Could you check a few things on this model? Use its own coordinates, in mm. A direction names the side the tool comes from. Coordinates: 2 decimals unless noted, no trailing zeros. Loops run counter-clockwise (first coordinate to the right, second up) from the corner with the lowest first, then second, coordinate; pieces in that order, holes last.
from build123d import *

# Parameters (mm, degrees)
F1_DEPTH = 8


with BuildPart() as f1:
    # F0 (on Front) → F1 (new body)
    with BuildSketch(Plane.XZ):
        Polygon((10.056205, -4.107465), (10.056205, -7.790019), (3.824189, -7.790019), (3.824189, -11.472573), (16.288221, -11.472573), (16.288221, -4.107465), align=None)
        with BuildLine():
            Line((3.824189, -11.472573), (3.824189, -7.790019))
            Line((3.824189, -7.790019), (-3.824189, -7.790019))
            Line((-3.824189, -7.790019), (-3.824189, -11.472573))
            Line((-3.824189, -11.472573), (-16.288221, -11.472573))
            ThreePointArc((-16.288221, -11.472573), (0, -27.760793), (16.288221, -11.472573))
            Line((16.288221, -11.472573), (3.824189, -11.472573))
        make_face()
        with BuildLine():
            Line((10.056205, 3.540918), (10.056205, -4.107465))
            Line((10.056205, -4.107465), (16.288221, -4.107465))
            ThreePointArc((16.288221, -4.107465), (20.112413, -0.283273), (16.288221, 3.540918))
            Line((16.288221, 3.540918), (10.056205, 3.540918))
        make_face()
        Polygon((-3.824189, -11.472573), (-3.824189, -7.790019), (-10.056205, -7.790019), (-10.056205, -4.107465), (-16.288221, -4.107465), (-16.288221, -11.472573), align=None)
        Polygon((10.056205, 7.790019), (10.056205, 3.540918), (16.288221, 3.540918), (16.288221, 12.039119), (3.824189, 12.039119), (3.824189, 7.790019), align=None)
        with BuildLine():
            Line((-16.288221, -4.107465), (-10.056205, -4.107465))
            Line((-10.056205, -4.107465), (-10.056205, 3.540918))
            Line((-10.056205, 3.540918), (-16.571494, 3.540918))
            ThreePointArc((-16.571494, 3.540918), (-20.115035, -0.419761), (-16.288221, -4.107465))
        make_face()
        with BuildLine():
            Line((-3.540916, 7.790019), (3.824189, 7.790019))
            Line((3.824189, 7.790019), (3.824189, 12.039119))
            Line((3.824189, 12.039119), (16.288221, 12.039119))
            ThreePointArc((16.288221, 12.039119), (-0.141636, 28.468977), (-16.571494, 12.039119))
            Line((-16.571494, 12.039119), (-3.540916, 12.039119))
            Line((-3.540916, 12.039119), (-3.540916, 7.790019))
        make_face()
        Polygon((-16.571494, 3.540918), (-10.056205, 3.540918), (-10.056205, 7.790019), (-3.540916, 7.790019), (-3.540916, 12.039119), (-16.571494, 12.039119), align=None)
    extrude(amount=F1_DEPTH)


solid = f1.part
(1) Which directions (+Z, -Z, +X, -X, +Y, -Y) give clear straight access to the entire face, cutting with the end or side of a thin tool? Please do faces 1 (the face through (16.288, -4, -8)), 2 (the face through (0, -4, -7.79)), 3 (the face through (-16.288, -4, -8)), 4 (the face through (16.288, -4, 8)), 5 (the face through (-0.358, -3.944, -27.757)).
Answers:
face 1: -Z, +X, +Y, -Y
face 2: +Y, -Y
face 3: -Z, -X, +Y, -Y
face 4: +Z, +X, +Y, -Y
face 5: -Z, +Y, -Y
(2) I need wall thicknesses on probe 1 along X at (y, z) = (-3, 0); probe 2 along X at (y, z) = (-5.25, 6); probe 3 along Z at (x, y) = (-4.5, -3.25). Which ranges of each line are inside material? Lowest first, please.
Answers:
probe 1: x = -20.11 to -10.06, 10.06 to 20.1
probe 2: x = -16.57 to -10.06, 10.06 to 16.29
probe 3: z = -27.13 to -7.79, 7.79 to 27.88
(3) For pin 1 (2 mm diameter, centred on y = -2, z = 2, fed in from -X); pin 2 (4 mm diameter, centred on y = -5.5, z = 7.5, fed in from -X); pin 3 (2 mm diameter, centred on x = -6.5, y = -5.5, fed in from -Z), each with a flat end and sliding along its axis, tell me the tip position at first contact or that it passes through.
Answers:
pin 1: stops at x = -19.9
pin 2: stops at x = -16.57
pin 3: stops at z = -26.8
(4) Imagine slicing it at A-A, the plane y = -5.25. Write out the boundary of the cut face in (x, z), and give its area (3 significant figures).
Answers:
outline: (-16.57, 3.54) arc R3.83 ccw to (-16.29, -4.11) - (-16.29, -11.47) arc R16.29 ccw to (16.29, -11.47) - (16.29, -4.11) arc R3.82 ccw to (16.29, 3.54) - (16.29, 12.04) arc R16.43 ccw to (-16.57, 12.04) - close; hole (-10.06, -7.79) - (10.06, -7.79) - (10.06, 7.79) - (-10.06, 7.79) - close
area: 1,340 mm2
(5) We'd pull the mould along X, two halves only. Please class faces 6 (the face through (-16.571, -4, 8)), 7 (the face through (0, 0, -12)), 8 (the face through (0.22, -3.944, 28.465)), 9 (the face through (0, -4, 7.79)): +X half, -X half, draft (parallel to the pull), parting line (faces both ways), or undercut.
Answers:
face 6: -X half
face 7: draft
face 8: parting line
face 9: undercut
(6) Imagine slicing it at D-D, the plane z = 9. Write out the boundary of the cut face in (x, y), and give its area (3 significant figures).
Answers:
outline: (-16.57, -8) - (16.29, -8) - (16.29, 0) - (-16.57, 0) - close
area: 263 mm2
(7) Imagine slicing it at C-C, the plane z = -6. Write out the boundary of the cut face in (x, y), and give its area (3 significant figures).
Answers:
outline: (-16.29, -8) - (-10.06, -8) - (-10.06, 0) - (-16.29, 0) - close; (10.06, -8) - (16.29, -8) - (16.29, 0) - (10.06, 0) - close
area: 99.7 mm2
(8) Imagine slicing it at B-B, the plane x = -5. Write out the boundary of the cut face in (y, z).
Answers:
outline: (-8, -26.97) - (0, -26.97) - (0, -7.79) - (-8, -7.79) - close; (-8, 7.79) - (0, 7.79) - (0, 27.73) - (-8, 27.73) - close
